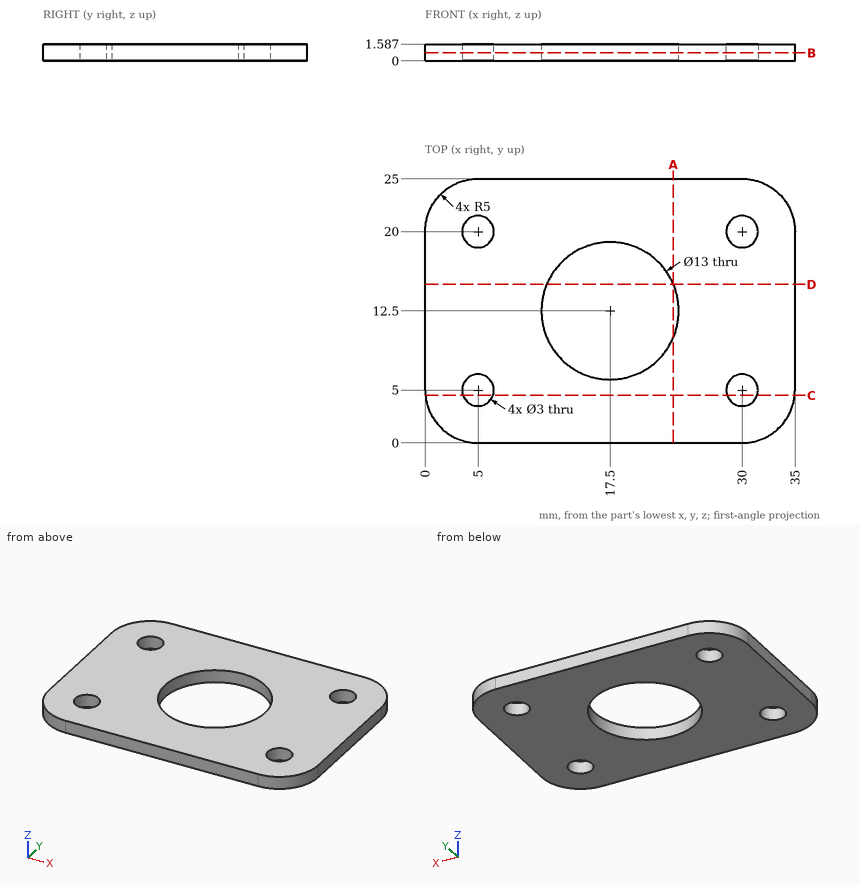
Answer from the drawing. Dimensions are ordinates in mm from the lowest x, y and z of the part. Give positions to 0.01 mm unless a question says otherwise; leave off trailing zeros. Write each loop counter-clockwise with the first axis right and the second up, starting at its lowest first coordinate (ties: lowest second). Pieces come first, ordered by that corner, then holes. Notation, with made-up numbers: (60.25, 74.5) -> (87.25, 74.5) arc R7 ccw to (87.25, 82.5) -> close; hole circle Ø2 at (5.25, 27.5). An arc over 180 degrees is marked (long way). Use a Markdown table: item, result.
(1) Section C-C, the plane y = 4.5 is taken. Determine the outline of the cut face in (x, z) (1 decimal).
Return value:
| item | result |
|---|---|
| outline | (0, 0) -> (3.6, 0) -> (3.6, 1.6) -> (0, 1.6) -> close; (6.4, 0) -> (28.6, 0) -> (28.6, 1.6) -> (6.4, 1.6) -> close; (31.4, 0) -> (35, 0) -> (35, 1.6) -> (31.4, 1.6) -> close |
(2) Find the intervals of material crossed by probe 1 along Y at (x, z) = (5, 0.4); probe 2 along Y at (x, z) = (17.5, 0.95); probe 3 along X at (y, z) = (3.75, 0.1) (1 decimal), in increasing order. Write a range as from..to.
Return value:
| item | result |
|---|---|
| probe 1 | 0..3.5, 6.5..18.5, 21.5..25 |
| probe 2 | 0..6, 19..25 |
| probe 3 | 0.2..4.2, 5.8..29.2, 30.8..34.8 |
(3) A flat-ended cylindrical pin translates along its axis: P1, Ø6, axis at x = 30.5, y = 21.5, coming from the -Z side. Find the tip coordinate at first contact, or state that the pin passes through.
Return value:
| item | result |
|---|---|
| P1 | z = 0 |
(4) Section D-D, the plane y = 15 is taken. Determine the outline of the cut face in (x, z).
Return value:
| item | result |
|---|---|
| outline | (0, 0) -> (11.5, 0) -> (11.5, 1.59) -> (0, 1.59) -> close; (23.5, 0) -> (35, 0) -> (35, 1.59) -> (23.5, 1.59) -> close |
(5) Section B-B, the plane z = 0.75 is taken. Determine the outline of the cut face in (x, y).
Return value:
| item | result |
|---|---|
| outline | (0, 5) arc R5 ccw to (5, 0) -> (30, 0) arc R5 ccw to (35, 5) -> (35, 20) arc R5 ccw to (30, 25) -> (5, 25) arc R5 ccw to (0, 20) -> close; hole circle Ø3 at (5, 5); hole circle Ø3 at (5, 20); hole circle Ø13 at (17.5, 12.5); hole circle Ø3 at (30, 5); hole circle Ø3 at (30, 20) |
(6) Section A-A, the plane x = 23.5 is taken. Determine the outline of the cut face in (y, z).
Return value:
| item | result |
|---|---|
| outline | (0, 0) -> (10, 0) -> (10, 1.59) -> (0, 1.59) -> close; (15, 0) -> (25, 0) -> (25, 1.59) -> (15, 1.59) -> close |
